from build123d import *

# Parameters (mm, degrees)
SKETCH1_W           = 220
SKETCH1_H           = 60
BOSS_EXTRUDE1_DEPTH = 20
FILLET1_R           = 3
SKETCH2_R           = 6
BOSS_EXTRUDE2_DEPTH = 20
SKETCH3_R           = 3.3
CUT_EXTRUDE1_DEPTH  = 20
SKETCH4_R           = 6
CUT_EXTRUDE2_DEPTH  = 15
FILLET2_R           = 3
FILLET3_R           = 3
FILLET4_R           = 3
FILLET6_R           = 3
FILLET7_R           = 3


with BuildPart() as part:
    # Sketch1 → Boss-Extrude1 (new body)
    with BuildSketch(Plane.XY):
        Rectangle(SKETCH1_W, SKETCH1_H)
    extrude(amount=BOSS_EXTRUDE1_DEPTH)

    # Fillet1
    fillet1_edges = [part.edges().sort_by_distance(p)[0] for p in [
        (110, -30, 10),
        (-110, -30, 10),
        (-110, 30, 10),
        (110, 30, 10),
    ]]
    fillet(fillet1_edges, radius=FILLET1_R)

    # Sketch2 → Boss-Extrude2 (add)
    with BuildSketch(Plane.XY.offset(20)):
        with Locations((-110, 0)):
            Circle(SKETCH2_R)
        with Locations((110, 0)):
            Circle(SKETCH2_R)
    extrude(amount=-BOSS_EXTRUDE2_DEPTH)

    # Sketch3 → Cut-Extrude1 (cut)
    with BuildSketch(Plane.XY.offset(20)):
        with Locations((-110, 0)):
            Circle(SKETCH3_R)
        with Locations((110, 0)):
            Circle(SKETCH3_R)
    extrude(amount=-CUT_EXTRUDE1_DEPTH, mode=Mode.SUBTRACT)

    # Sketch4 → Cut-Extrude2 (cut)
    with BuildSketch(Plane.XY.offset(20)):
        with Locations((-110, 0)):
            Circle(SKETCH4_R)
        with Locations((110, 0)):
            Circle(SKETCH4_R)
    extrude(amount=-CUT_EXTRUDE2_DEPTH, mode=Mode.SUBTRACT)

    # Fillet2
    fillet2_edges = [part.edges().sort_by_distance(p)[0] for p in [
        (-110, 6, 2.5),
        (-110, -6, 2.5),
    ]]
    fillet(fillet2_edges, radius=FILLET2_R)

    # Fillet3
    fillet3_edges = [part.edges().sort_by_distance(p)[0] for p in [
        (-110, 6, 12.5),
    ]]
    fillet(fillet3_edges, radius=FILLET3_R)

    # Fillet4
    fillet4_edges = [part.edges().sort_by_distance(p)[0] for p in [
        (-110, -6, 12.5),
    ]]
    fillet(fillet4_edges, radius=FILLET4_R)

    # Fillet6
    fillet6_edges = [part.edges().sort_by_distance(p)[0] for p in [
        (110, -6, 2.5),
        (110, 6, 2.5),
    ]]
    fillet(fillet6_edges, radius=FILLET6_R)

    # Fillet7
    fillet7_edges = [part.edges().sort_by_distance(p)[0] for p in [
        (110, 6, 12.5),
        (110, -6, 12.5),
    ]]
    fillet(fillet7_edges, radius=FILLET7_R)


solid = part.part
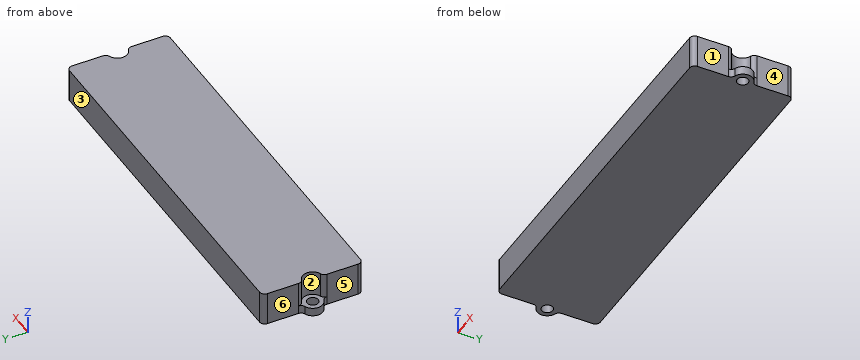
Verification items for the finished model (mm, model axes). Face numbers are marked on the shaded views. A direction names the side the tool comes from. Round coordinates to 2 decimals unless told otherwise and drop trailing zeros. Loops run counter-clockwise (first coordinate to the right, second up) from the corner with the lowest first, then second, coordinate; pieces in that order, holes last. Notation, with made-up numbers: (23, 80.5) - (52, 80.5) arc R29 ccw to (52, 101.5) - close; hole circle Ø1 at (-36, 21). An arc over 180 degrees is marked (long way). Use one line per item in the form item = value.
1. Draft check along Y on the marked faces 1, 2 and 3. Enter one of: pulls with the +Y half, pulls with the -Y half, needs draft (parallel to the pull), parting line crosses it, or undercut.
A:
face_1 = needs draft
face_2 = undercut
face_3 = pulls with the +Y half
2. Section check B-B on z = 13.25. Record the cut outline in (x, y).
A:
outline = (-110, -27) arc R3 ccw to (-107, -30) - (107, -30) arc R3 ccw to (110, -27) - (110, -8.49) arc R3 ccw to (108, -5.66) arc R6 cw to (108, 5.66) arc R3 ccw to (110, 8.49) - (110, 27) arc R3 ccw to (107, 30) - (-107, 30) arc R3 ccw to (-110, 27) - (-110, 8.49) arc R3 ccw to (-108, 5.66) arc R6 cw to (-108, -5.66) arc R3 ccw to (-110, -8.49) - close
3. Section check C-C on y = -22. Record the cut outline in (x, z), and give its area (3 significant figures).
A:
outline = (-110, 0) - (110, 0) - (110, 20) - (-110, 20) - close
area = 4,400 mm²
4. Access from +Z, -Z, +X, -X, +Y, -Y to the whole of each face (thin tool, end or side, straight path). Record for the marked faces 4, 5 and 6.
A:
face_4 = +Z, -Z, +X, +Y
face_5 = +Z, -Z, -X, -Y
face_6 = +Z, -Z, -X, +Y
5. Scan lines: probe 1 along X at (y, z) = (-16, 16.75); probe 2 along X at (y, z) = (-4.5, 9.5). Record each from-to range of solid material in increasing order.
A:
probe_1 = -110 to 110
probe_2 = -106.03 to 106.03
6. Section check A-A on y = 0. Record the cut outline in (x, z).
A:
outline = (-116, 0) - (-113.3, 0) - (-113.3, 5) - (-116, 5) - close; (-106.7, 0) - (106.7, 0) - (106.7, 5) - (104, 5) - (104, 20) - (-104, 20) - (-104, 5) - (-106.7, 5) - close; (113.3, 0) - (116, 0) - (116, 5) - (113.3, 5) - close
7. Gauge pin test, flat ends, axial feed: pin 1 Ø6 at (x, y) = (-110.5, -0.5) entering from +Z; pin 2 Ø5 at (y, z) = (-11.5, 7.5) entering from -X; pin 3 Ø9.5 at (y, z) = (-16.5, 13) entering from +X. Record the tip position at first contact, or that the pin passes through.
A:
pin_1 = 5
pin_2 = -110
pin_3 = 110
